Autodesk Inventor part; units mm, degrees
ref_plane "YZ Plane" through (0, 0, 0) normal (1, 0, 0) x (0, 1, 0)
ref_plane "XZ Plane" through (0, 0, 0) normal (0, 1, 0) x (-1, 0, 0)
ref_plane "XY Plane" through (0, 0, 0) normal (0, 0, 1) x (1, 0, 0)
sketch "Sketch1" plane through (0, 0, 0) normal (0, 1, 0) x (-1, 0, 0)
  line L0 (-8.75, 22) -> (-8.75, -22)
  line L1 (-8.75, -22) -> (8.75, -22)
  line L2 (8.75, -22) -> (8.75, 22)
  line L3 (8.75, 22) -> (-8.75, 22)
  line L4 (-8.75, 22) -> (8.75, -22) construction
  line L5 (-8.75, -22) -> (8.75, 22) construction
  line L6 (-8.75, 22) -> (-1.75, 22)
  point P0 (0, 0)
  dimension "d1" = 44
  dimension "d2" = 17.5
extrude "Extrusion1" add sketch "Sketch1" along normal blind 2
sketch "Sketch2" plane through (0, 2, 0) normal (0, 1, 0) x (1, 0, 0)
  line L0 (8.75, 22) -> (-8.75, 22)
  line L1 (-8.6195, 22) -> (8.6907, 22) construction
  line L2 (8.6907, 22) -> (8.6907, -23.9682) construction
  line L3 (8.6907, -23.9682) -> (-8.6195, -23.9682) construction
  line L4 (-8.6195, -23.9682) -> (-8.6195, 22) construction
  circle A0 centre (0.05, -5.1) radius 1.5
  line L5 (8.75, -22) -> (8.75, 22)
  line L6 (-8.75, -22) -> (8.75, -22)
  point P0 (0, 0)
  dimension "d39" = 3
  dimension "d42" = 8.7
  dimension "d43" = 16.9
decal "Decal1"
sketch "Sketch3" plane through (0, 2, 0) normal (0, 1, 0) x (1, 0, 0)
  circle A0 centre (0.05, -5.1) radius 1.5
  line L0 (8.75, -22) -> (8.75, -101.371)
  line L1 (-21.6488, -22) -> (8.75, -22)
  line L2 (8.75, -22) -> (8.75, 22)
  line L3 (-8.75, -22) -> (8.75, -22)
  point P0 (0, 0)
  point P1 (-12.8988, -61.6855)
  dimension "d44" = 3
  dimension "d45" = 8.7
  dimension "d46" = 16.9
extrude "Extrusion2" cut sketch "Sketch3" against normal through all
sketch "Sketch4" plane through (0, 2, 0) normal (0, 1, 0) x (1, 0, 0)
  line L0 (4.75, 20.5) -> (3.75, 20.5)
  line L1 (3.75, 20.5) -> (3.75, 28)
  line L2 (3.75, 28) -> (4.75, 28)
  line L3 (4.75, 28) -> (4.75, 20.5)
  line L4 (8.75, -22) -> (8.75, 22)
  line L5 (8.75, 22) -> (-8.75, 22)
  point P0 (0, 0)
  dimension "d51" = 4
  dimension "d52" = 1
  dimension "d53" = 1.5
  dimension "d54" = 7.5
extrude "Extrusion3" add sketch "Sketch4" along normal blind 3
properties part number "3DModel"
Verification items for the finished model (mm, model axes). A direction names the side the tool comes from. Round coordinates to 2 decimals unless told otherwise and drop trailing zeros. Write each loop counter-clockwise with the first axis right and the second up, starting at its lowest first coordinate (ties: lowest second). Pieces come first, ordered by that corner, then holes.
(1) Section check C-C (x = -5.75). Enter the section's corners in (y, z), plus the area to 3 significant figures.
Returned:
outline: (0, -22) - (2, -22) - (2, 22) - (0, 22) - close
area: 88.0 mm2
(2) Section check B-B (z = 5.1). Enter the section's corners in (x, y), plus the area to 3 significant figures.
Returned:
outline: (-8.75, 0) - (-1.45, 0) - (-1.45, 2) - (-8.75, 2) - close; (1.55, 0) - (8.75, 0) - (8.75, 2) - (1.55, 2) - close
area: 29.0 mm2
(3) Depth check by flat-ended pin: pin 1 Ø2.5 at (y, z) = (3, -26) entering from -X; pin 2 Ø3 at (x, y) = (5, 4) entering from -Z; pin 3 Ø0.6 at (x, y) = (1, 1) entering from -Z; pin 4 Ø3 at (x, y) = (-3, 4.5) entering from -Z. Enter the tip coordinate at first touch or a pass-through.
Returned:
pin 1: stops at x = 3.75
pin 2: stops at z = -28
pin 3: stops at z = -22
pin 4: passes through
(4) Section check D-D (y = 2.9). Enter the section's corners in (x, z), plus the area to 3 significant figures.
Returned:
outline: (3.75, -28) - (4.75, -28) - (4.75, -20.5) - (3.75, -20.5) - close
area: 7.50 mm2
(5) Mould release check, pull along Z, two halves, no side actions. Record for faces 4 (the flat face through (0, 1, -22)), 5 (the flat face through (4, 5, -24)), 6 (the flat face through (4, 3, -20.5)), 7 (the cylindrical face through (-1.14, 1.01, 6.01)): pulls with the +Z half, pulls with the -Z half, needs draft (parallel to the pull), parting line crosses it, or undercut.
Returned:
face 4: pulls with the -Z half
face 5: needs draft
face 6: pulls with the +Z half
face 7: undercut
(6) Material ranges on line 1 (Z direction, x = 0.05, y = 1.2); line 2 (X direction, y = 0.6, z = 5.1); line 3 (Y direction, x = 7.25, z = 13.5), recorded low to high.
Returned:
line 1: z = -22 to 3.6, 6.6 to 22
line 2: x = -8.75 to -1.45, 1.55 to 8.75
line 3: y = 0 to 2
(7) Section check A-A (x = 0.05). Enter the section's corners in (y, z).
Returned:
outline: (0, -22) - (2, -22) - (2, 3.6) - (0, 3.6) - close; (0, 6.6) - (2, 6.6) - (2, 22) - (0, 22) - close
(8) Access from +Z, -Z, +X, -X, +Y, -Y to the whole of each face (thin tool, end or side, straight path). Record for faces 1 (the flat face through (3.75, 3, -24)), 2 (the flat face through (4.75, 3, -24)), 3 (the flat face through (4, 2, -25)).
Returned:
face 1: +Z, -Z, -X, +Y
face 2: +Z, -Z, +X, +Y
face 3: -Z, +X, -X, -Y
